Geometry: final body of the model. Coordinates: model frame, mm. A direction names the side the tool comes from. Round coordinates to 2 decimals unless told otherwise and drop trailing zeros. Loops run counter-clockwise (first coordinate to the right, second up) from the corner with the lowest first, then second, coordinate; pieces in that order, holes last. Notation, with made-up numbers: (5, -10) - (62, -10) arc R17 cw to (62, 6) - close; hole circle Ø4 at (82.25, -33.5). An arc over 180 degrees is marked (long way). Answer as CSV lines item,"result".
from build123d import *

# Parameters (mm, degrees)
BOSS_EXTRUDE1_DEPTH   = 5
BOSS_EXTRUDE1_2_DEPTH = 5
BOSS_EXTRUDE1_3_DEPTH = 5
BOSS_EXTRUDE1_4_DEPTH = 5
SKETCH2_W             = 55
SKETCH2_H             = 50
BOSS_EXTRUDE2_DEPTH   = 5
SKETCH3_W             = 55
SKETCH3_H             = 13
SKETCH3_R             = 2.1
BOSS_EXTRUDE3_DEPTH   = 5
SKETCH4_W             = 61
SKETCH4_H             = 30
BOSS_EXTRUDE4_DEPTH   = 5
SKETCH5_R             = 2.5
SKETCH5_W             = 39.983210939
SKETCH5_H             = 20
CUT_EXTRUDE3_DEPTH    = 5
SKETCH7_R             = 2.1
CUT_EXTRUDE4_DEPTH    = 14


with BuildPart() as part:
    # Sketch1 → Boss-Extrude1 (new body)
    with BuildSketch(Plane.XY):
        with BuildLine():
            Line((23.840984083, 9.134098408), (28.840984083, 9.134098408))
            Line((28.840984083, 9.134098408), (28.840984083, 25.134098408))
            Line((28.840984083, 25.134098408), (19.840984083, 25.134098408))
            Line((19.840984083, 25.134098408), (19.840984083, 13.134098408))
            ThreePointArc((19.840984083, 13.134098408), (21.012556959, 10.305671284), (23.840984083, 9.134098408))
        make_face()
    extrude(amount=BOSS_EXTRUDE1_DEPTH)



with BuildPart() as body_2:
    # Sketch1 → Boss-Extrude1 2 (new body)
    with BuildSketch(Plane.XY):
        with BuildLine():
            Line((-26.159015917, 9.134098408), (-21.159015917, 9.134098408))
            ThreePointArc((-21.159015917, 9.134098408), (-18.330588792, 10.305671284), (-17.159015917, 13.134098408))
            Line((-17.159015917, 13.134098408), (-17.159015917, 25.134098408))
            Line((-17.159015917, 25.134098408), (-26.159015917, 25.134098408))
            Line((-26.159015917, 25.134098408), (-26.159015917, 9.134098408))
        make_face()
    extrude(amount=BOSS_EXTRUDE1_2_DEPTH)


with BuildPart() as body_3:
    # Sketch1 → Boss-Extrude1 3 (new body)
    with BuildSketch(Plane.XY):
        with BuildLine():
            Line((28.840984083, -8.865901592), (23.840984083, -8.865901592))
            ThreePointArc((23.840984083, -8.865901592), (21.012556959, -10.037474467), (19.840984083, -12.865901592))
            Line((19.840984083, -12.865901592), (19.840984083, -24.865901592))
            Line((19.840984083, -24.865901592), (28.840984083, -24.865901592))
            Line((28.840984083, -24.865901592), (28.840984083, -8.865901592))
        make_face()
    extrude(amount=BOSS_EXTRUDE1_3_DEPTH)


with BuildPart() as body_4:
    # Sketch1 → Boss-Extrude1 4 (new body)
    with BuildSketch(Plane.XY):
        with BuildLine():
            Line((-17.159015917, -24.865901592), (-17.159015917, -12.865901592))
            ThreePointArc((-17.159015917, -12.865901592), (-18.330588792, -10.037474467), (-21.159015917, -8.865901592))
            Line((-21.159015917, -8.865901592), (-26.159015917, -8.865901592))
            Line((-26.159015917, -8.865901592), (-26.159015917, -24.865901592))
            Line((-26.159015917, -24.865901592), (-17.159015917, -24.865901592))
        make_face()
    extrude(amount=BOSS_EXTRUDE1_4_DEPTH)


with BuildPart() as part_1:
    add(part.part)

    add(body_2.part)  # Boss-Extrude2 merges body 2

    add(body_3.part)  # Boss-Extrude2 merges body 3

    add(body_4.part)  # Boss-Extrude2 merges body 4
    # Sketch2 → Boss-Extrude2 (add)
    with BuildSketch(Plane.XY.offset(5)):
        with Locations((1.340984083, 0.134098408)):
            Rectangle(SKETCH2_W, SKETCH2_H)
    extrude(amount=BOSS_EXTRUDE2_DEPTH)

    # Sketch3 → Boss-Extrude3 (add)
    with BuildSketch(Plane(origin=(0, 25.134098408, 0), x_dir=(1, 0, 0), z_dir=(0, 1, 0))):
        with Locations((1.340984083, -3.5)):
            Rectangle(SKETCH3_W, SKETCH3_H)
        with Locations((-8.659015917, -1)):
            Circle(SKETCH3_R, mode=Mode.SUBTRACT)
        with Locations((11.340984083, -1)):
            Circle(SKETCH3_R, mode=Mode.SUBTRACT)
    boss_extrude3 = extrude(amount=BOSS_EXTRUDE3_DEPTH)

    # Mirror1: Boss-Extrude3 across plane
    add(boss_extrude3.mirror(Plane(origin=(0, 0.134098408, 0), x_dir=(0, 0, 1), z_dir=(0, -1, 0))))

    # Sketch4 → Boss-Extrude4 (add)
    with BuildSketch(Plane(origin=(0, 30.134098408, 0), x_dir=(1, 0, 0), z_dir=(0, 1, 0))):
        with Locations((1.340984083, -25)):
            Rectangle(SKETCH4_W, SKETCH4_H)
    boss_extrude4 = extrude(amount=-BOSS_EXTRUDE4_DEPTH)

    # Mirror2: Boss-Extrude4 across plane
    add(boss_extrude4.mirror(Plane(origin=(0, 0.134098408, 0), x_dir=(0, 0, 1), z_dir=(0, -1, 0))))

    # Sketch5 → Cut-Extrude3 (cut)
    with BuildSketch(Plane.XZ.offset(-25.134098408)):
        with Locations((-23.159015917, 29.025922811)):
            Circle(SKETCH5_R)
        with Locations((-23.159015917, 18.865922811)):
            Circle(SKETCH5_R)
        with Locations((25.840984083, 29.025922811)):
            Circle(SKETCH5_R)
        with Locations((25.840984083, 18.865922811)):
            Circle(SKETCH5_R)
        with Locations((1.332589552, 23.945922811)):
            Rectangle(SKETCH5_W, SKETCH5_H)
    cut_extrude3 = extrude(amount=-CUT_EXTRUDE3_DEPTH, mode=Mode.SUBTRACT)

    # Sketch7 → Cut-Extrude4 (cut, through all)
    with BuildSketch(Plane.XY.offset(10)):
        with Locations((23.840984083, -12.865901592)):
            Circle(SKETCH7_R)
        with Locations((-21.159015917, -12.865901592)):
            Circle(SKETCH7_R)
        with Locations((23.840984083, 13.134098408)):
            Circle(SKETCH7_R)
        with Locations((-21.159015917, 13.134098408)):
            Circle(SKETCH7_R)
    extrude(amount=-CUT_EXTRUDE4_DEPTH, mode=Mode.SUBTRACT)

    # Mirror3: Cut-Extrude3 across plane
    add(cut_extrude3.mirror(Plane(origin=(0, 0.134098408, 0), x_dir=(0, 0, 1), z_dir=(0, -1, 0))), mode=Mode.SUBTRACT)


solid = part_1.part
(1) Section D-D (x = 8). Output: boundary loops of the cut face in (y, z), and give its area (3 significant figures).
Findings below:
outline,"(-29.87, -3) - (-24.87, -3) - (-24.87, 5) - (25.13, 5) - (25.13, -3) - (30.13, -3) - (30.13, 13.95) - (25.13, 13.95) - (25.13, 10) - (-24.87, 10) - (-24.87, 13.95) - (-29.87, 13.95) - close; (-29.87, 33.95) - (-24.87, 33.95) - (-24.87, 40) - (-29.87, 40) - close; (25.13, 33.95) - (30.13, 33.95) - (30.13, 40) - (25.13, 40) - close"
area,"480 mm2"
(2) Section C-C (z = 23). Output: boundary loops of the cut face in (x, y).
Findings below:
outline,"(-29.16, -29.87) - (-18.66, -29.87) - (-18.66, -24.87) - (-29.16, -24.87) - close; (-29.16, 25.13) - (-18.66, 25.13) - (-18.66, 30.13) - (-29.16, 30.13) - close; (21.32, -29.87) - (31.84, -29.87) - (31.84, -24.87) - (21.32, -24.87) - close; (21.32, 25.13) - (31.84, 25.13) - (31.84, 30.13) - (21.32, 30.13) - close"
(3) Draft query along Z for faces 4 (the face through (1, -27, 40)), 5 (the face through (-23.257, 13.226, 5.07)), 6 (the face through (-21.815, 27.599, 31.134)). Return one class per face: pulls with the +Z half, pulls with the -Z half, needs draft (parallel to the pull), parting line crosses it, or undercut.
Findings below:
face 4,"pulls with the +Z half"
face 5,"needs draft"
face 6,"undercut"
(4) Section A-A (z = 36). Output: boundary loops of the cut face in (x, y).
Findings below:
outline,"(-29.16, -29.87) - (31.84, -29.87) - (31.84, -24.87) - (-29.16, -24.87) - close; (-29.16, 25.13) - (31.84, 25.13) - (31.84, 30.13) - (-29.16, 30.13) - close"
(5) Section B-B (x = -7.5). Output: boundary loops of the cut face in (y, z), and give its area (3 significant figures).
Findings below:
outline,"(-29.87, -3) - (-24.87, -3) - (-24.87, -0.75) - (-29.87, -0.75) - close; (-29.87, 2.75) - (-24.87, 2.75) - (-24.87, 5) - (25.13, 5) - (25.13, 2.75) - (30.13, 2.75) - (30.13, 13.95) - (25.13, 13.95) - (25.13, 10) - (-24.87, 10) - (-24.87, 13.95) - (-29.87, 13.95) - close; (-29.87, 33.95) - (-24.87, 33.95) - (-24.87, 40) - (-29.87, 40) - close; (25.13, -3) - (30.13, -3) - (30.13, -0.75) - (25.13, -0.75) - close; (25.13, 33.95) - (30.13, 33.95) - (30.13, 40) - (25.13, 40) - close"
area,"445 mm2"
(6) Material intervals for line 1 along Y through (x, z) = (11.5, 37); line 2 along X through (y, z) = (27.95, 1); line 3 along Y through (x, z) = (-22.5, 3.5), sorted ascending.
Findings below:
line 1,"-29.87 to -24.87, 25.13 to 30.13"
line 2,"-26.16 to -10.76, -6.56 to 9.24, 13.44 to 28.84"
line 3,"-29.87 to -14.48, -11.25 to -8.87, 9.13 to 11.52, 14.75 to 30.13"
(7) Access query for faces 1 (the face through (19.841, -19, 2)), 2 (the face through (24, 17, 0)), 3 (the face through (1, 28, 33.946)). Directions: +Z, -Z, +X, -X, +Y, -Y. A direction counts if a zero-diameter tool reaches every point of the face in a straight line with its end or side. Return the directions, or none.
Findings below:
face 1,"-Z"
face 2,"-Z, +X, -X"
face 3,"+Y, -Y"
(8) Pin query (flat end, axial travel): P1, Ø3.5, axis at x = 23.84, y = -12.87, coming from the -Z side; P2, Ø2.5, axis at x = -27.5, y = -27, coming from the -Z side; P3, Ø2.5, axis at x = -19.5, y = 17.5, coming from the -Z side; P4, Ø15, axis at x = -8, y = 8, coming from the -Z side. Return the tip coordinate at first contact, or that it passes through.
Findings below:
P1,"through"
P2,"z = 10"
P3,"z = 0"
P4,"z = 5"
